Verification items for this drawing (mm, ordinates from the low corner). Round coordinates to 2 decimals unless told otherwise and drop trailing zeros. Order: outer loops, then holes, each group sorted by start corner. A loop starts at its lowest first (then second) coordinate and runs counter-clockwise, first axis right, second up. Notation, with made-up numbers: (-37.5, 59.5) - (-20.5, 59.5) arc R22 ccw to (-20.5, 98.5) - close; hole circle Ø11 at (-25, -25). An arc over 180 degrees is marked (long way). Use a Markdown table: item, result. Add a question column.
(1) Section check A-A on x = 50.8. Record the boundary of the cut face in (y, z) (3 decimals).
(2) Section check B-B on y = 12.7. Record the boundary of the cut face in (x, z) (3 decimals), then the cut area to 3 significant figures.
(3) Gauge pin test, flat ends, axial feed: P1, Ø1, axis at y = 69.5, z = 8, coming from the +X side; P2, Ø5, axis at x = 12.7, y = 88.9, coming from the +Z side; P3, Ø3, axis at y = 29, z = 7, coming from the +X side; P4, Ø3, axis at x = 99.5, y = 43, coming from the +Z side (3 decimals). Record the tip position at first contact, or that the pin passes through.
(4) Thickness scan on line 1 along X through (y, z) = (90.5, 7.5); line 2 along X through (y, z) = (74, 8.75); line 3 along Y through (x, z) = (81.5, 7.75) (1 decimal). Record the ranges inside material, lowest first. Write a range as [from, to].
(5) Section check C-C on y = 50.8. Record the boundary of the cut face in (x, z) (3 decimals).
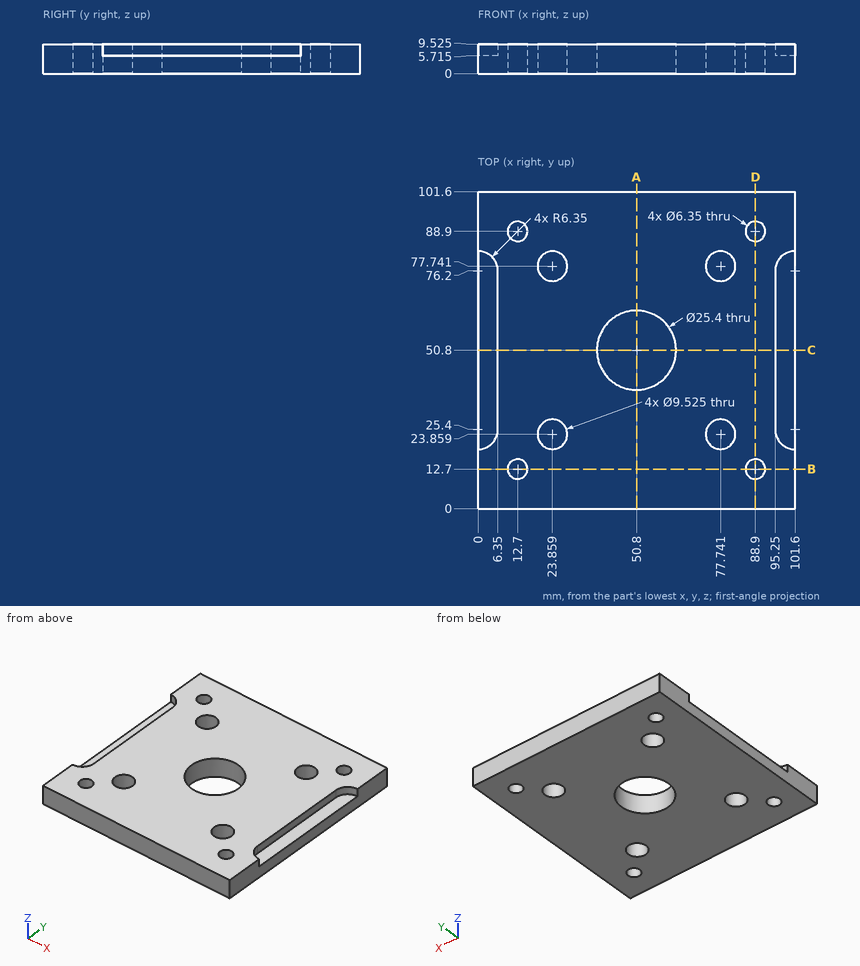
Check sheet entries:
| question | item | result |
|---|---|---|
| 1 | outline | (0, 0) - (38.1, 0) - (38.1, 9.525) - (0, 9.525) - close; (63.5, 0) - (101.6, 0) - (101.6, 9.525) - (63.5, 9.525) - close |
| 2 | outline | (0, 0) - (9.525, 0) - (9.525, 9.525) - (0, 9.525) - close; (15.875, 0) - (85.725, 0) - (85.725, 9.525) - (15.875, 9.525) - close; (92.075, 0) - (101.6, 0) - (101.6, 9.525) - (92.075, 9.525) - close |
| 2 | area | 847 mm2 |
| 3 | P1 | stops at x = 95.25 |
| 3 | P2 | passes through |
| 3 | P3 | stops at x = 101.6 |
| 3 | P4 | stops at z = 5.715 |
| 4 | line 1 | x = [0, 9.96], [15.44, 86.16], [91.64, 101.6] |
| 4 | line 2 | x = [6.35, 20.91], [26.81, 74.79], [80.69, 95.25] |
| 4 | line 3 | y = [0, 20.9], [26.8, 74.8], [80.7, 101.6] |
| 5 | outline | (0, 0) - (38.1, 0) - (38.1, 9.525) - (6.35, 9.525) - (6.35, 5.715) - (0, 5.715) - close; (63.5, 0) - (101.6, 0) - (101.6, 5.715) - (95.25, 5.715) - (95.25, 9.525) - (63.5, 9.525) - close |
